from build123d import *

# Parameters (mm, degrees)
F0_W     = 15
F0_H     = 30
F1_DEPTH = 150
F2_R     = 5.08
F3_R     = 5.08


with BuildPart() as f1:
    # F0 (on Top) → F1 (new body)
    with BuildSketch(Plane.XY):
        with Locations((-0.622407, 7.366808)):
            Rectangle(F0_W, F0_H)
    extrude(amount=F1_DEPTH)

    # F2
    f2_edges = [f1.edges().sort_by_distance(p)[0] for p in [
        (6.877593, -7.633192, 75),
        (6.877593, 7.366808, 0),
    ]]
    fillet(f2_edges, radius=F2_R)

    # F3
    f3_edges = [f1.edges().sort_by_distance(p)[0] for p in [
        (6.877593, 9.906808, 150),
    ]]
    fillet(f3_edges, radius=F3_R)


solid = f1.part
The listing builds one solid part. Answer for the finished solid, in the listing's coordinates (mm). Coordinates: 2 decimals unless noted, no trailing zeros. Loops run counter-clockwise (first coordinate to the right, second up) from the corner with the lowest first, then second, coordinate; pieces in that order, holes last.
1) A flat-ended cylindrical pin translates along its axis: pin 1 Ø1.5 at (x, y) = (4.5, 1.5) entering from -Z. Find the tip coordinate at first contact, or state that the pin passes through.
2) Find section A-A on x = 4. Write down the section's boundary in (y, z), then the cut area to 3 significant figures.
3) Find the intervals of material crossed by L1, parallel to Z at x = -0.5, y = -2.75; L2, parallel to Z at x = -1.75, y = -3.75; L3, parallel to Y at x = 3.5, z = 105, in increasing order.
Values:
1. pin 1: stops at z = 0.39
2. outline: (-7.13, 0.5) - (22.37, 0.5) - (22.37, 149.5) - (-2.55, 149.5) arc R4.58 ccw to (-7.13, 144.92) - close
2. area: 4,390 mm2
3. L1: z = 0 to 150
3. L2: z = 0 to 149.86
3. L3: y = -7.34 to 22.37
